from build123d import *

# Parameters (mm, degrees)
F0_R      = 60
F1_DEPTH  = 40
F3_R      = 10
F2_R      = 40
F4_DEPTH  = 4
F5_R      = 40
F6_DEPTH  = 4
F7_R      = 11
F8_DEPTH  = 7
F9_R      = 11
F10_DEPTH = 7
F12_D     = 10


with BuildPart() as f1:
    # F0 (on Front) → F1 (new body)
    with BuildSketch(Plane.XZ):
        Circle(F0_R)
    extrude(amount=F1_DEPTH)

    # F3
    f3_edges = [f1.edges().sort_by_distance(p)[0] for p in [
        (-60, 0, 0),
        (60, -20, 0),
        (-60, -40, 0),
    ]]
    fillet(f3_edges, radius=F3_R)

    # F2 (on face) → F4 (cut)
    with BuildSketch(Plane.XZ.offset(40)):
        Circle(F2_R)
    extrude(amount=-F4_DEPTH, mode=Mode.SUBTRACT)

    # F5 (on face) → F6 (cut)
    with BuildSketch(Plane(origin=(0, 0, 0), x_dir=(-1, 0, 0), z_dir=(0, 1, 0))):
        Circle(F5_R)
    extrude(amount=-F6_DEPTH, mode=Mode.SUBTRACT)

    # F7 (on face) → F8 (cut)
    with BuildSketch(Plane(origin=(0, -4, 0), x_dir=(-1, 0, 0), z_dir=(0, 1, 0))):
        Circle(F7_R)
    extrude(amount=-F8_DEPTH, mode=Mode.SUBTRACT)

    # F9 (on face) → F10 (cut)
    with BuildSketch(Plane.XZ.offset(36)):
        Circle(F9_R)
    extrude(amount=-F10_DEPTH, mode=Mode.SUBTRACT)

    # F12 (through all)
    with Locations(Plane(origin=(0, -4, 0), x_dir=(-1, 0, 0), z_dir=(0, 1, 0))):
        with Locations((0, 0)):
            Hole(F12_D / 2)


solid = f1.part
The model under review builds one solid part; all positions refer to its coordinate system, in mm. A direction names the side the tool comes from. Coordinates: 2 decimals unless noted, no trailing zeros. Write each loop counter-clockwise with the first axis right and the second up, starting at its lowest first coordinate (ties: lowest second). Pieces come first, ordered by that corner, then holes. Notation, with made-up numbers: (-13, 78) -> (27, 78) arc R7 cw to (27, 82) -> close; hole circle Ø6 at (20, 28). An arc over 180 degrees is marked (long way). Answer in a Markdown table with one row per item.
1. We need section C-C, the plane y = -20. State the section outline as (x, z) points.
Answers below:
| item | result |
|---|---|
| outline | circle Ø120 at (0, 0); hole circle Ø10 at (0, 0) |
2. We need section B-B, the plane x = 0. State the section outline as (y, z) points, and give its area (3 significant figures).
Answers below:
| item | result |
|---|---|
| outline | (-40, -50) arc R10 ccw to (-30, -60) -> (-10, -60) arc R10 ccw to (0, -50) -> (0, -40) -> (-4, -40) -> (-4, -11) -> (-11, -11) -> (-11, -5) -> (-29, -5) -> (-29, -11) -> (-36, -11) -> (-36, -40) -> (-40, -40) -> close; (-40, 40) -> (-36, 40) -> (-36, 11) -> (-29, 11) -> (-29, 5) -> (-11, 5) -> (-11, 11) -> (-4, 11) -> (-4, 40) -> (0, 40) -> (0, 50) arc R10 ccw to (-10, 60) -> (-30, 60) arc R10 ccw to (-40, 50) -> close |
| area | 3,590 mm^2 |
3. Draft analysis for pull direction X (two halves, no side actions). For faces 4 (the cylindrical face through (-59.94, -19.86, 2.64)), 5 (the flat face through (-22, -40, 34)), 6 (the flat face through (-8, -4, -8)), state which applies: +X half, -X half, draft (parallel to the pull), parting line (faces both ways), or undercut.
Answers below:
| item | result |
|---|---|
| face 4 | parting line |
| face 5 | draft |
| face 6 | undercut |
4. For faces 1 (the cylindrical face through (-8.67, -38.03, -39.05)), 2 (the cylindrical face through (-1.08, -20.13, -4.88)), 3 (the cylindrical face through (2.38, -7.45, -10.74)), list the 3-axis set-ups (+Z, -Z, +X, -X, +Y, -Y) from which the entire face can be reached by the end or side of a thin tool; tool diameter is ignored.
Answers below:
| item | result |
|---|---|
| face 1 | -Y |
| face 2 | +Y, -Y |
| face 3 | +Y |
5. Wall thickness on probe 1 along Y at (x, z) = (-34, 21); probe 2 along Z at (x, y) = (0, -32); probe 3 along Z at (x, y) = (0, -33.5): over which ranges is each line inside the solid? List them lowest first. Write a range as [from, to].
Answers below:
| item | result |
|---|---|
| probe 1 | y = [-36, -4] |
| probe 2 | z = [-59.8, -11], [11, 59.8] |
| probe 3 | z = [-59.37, -11], [11, 59.37] |
6. We need section D-D, the plane y = -8. State the section outline as (x, z) points.
Answers below:
| item | result |
|---|---|
| outline | circle Ø119.6 at (0, 0); hole circle Ø22 at (0, 0) |
7. Clearance check with flat-ended pins moving along their axes: pin 1 Ø17.5 at (x, z) = (-5, 4) entering from +Y; pin 2 Ø24 at (x, z) = (2.5, -1) entering from -Y; pin 3 Ø1.5 at (x, z) = (46, -41.5) entering from +Y; pin 4 Ø5 at (x, y) = (10, -9) entering from +Z. State where each tip first meets the part, or that it passes through.
Answers below:
| item | result |
|---|---|
| pin 1 | stops at y = -4 |
| pin 2 | stops at y = -36 |
| pin 3 | passes through |
| pin 4 | stops at z = 59.51 |
8. We need section A-A, the plane z = 0. State the section outline as (x, y) points, and give its area (3 significant figures).
Answers below:
| item | result |
|---|---|
| outline | (-60, -30) arc R10 ccw to (-50, -40) -> (-40, -40) -> (-40, -36) -> (-11, -36) -> (-11, -29) -> (-5, -29) -> (-5, -11) -> (-11, -11) -> (-11, -4) -> (-40, -4) -> (-40, 0) -> (-50, 0) arc R10 ccw to (-60, -10) -> close; (5, -29) -> (11, -29) -> (11, -36) -> (40, -36) -> (40, -40) -> (50, -40) arc R10 ccw to (60, -30) -> (60, -10) arc R10 ccw to (50, 0) -> (40, 0) -> (40, -4) -> (11, -4) -> (11, -11) -> (5, -11) -> close |
| area | 3,590 mm^2 |
